Build history of the part. All positions in model axes, mm. A direction names the side the tool comes from. Coordinates: 2 decimals unless noted, no trailing zeros. Write each loop counter-clockwise with the first axis right and the second up, starting at its lowest first coordinate (ties: lowest second). Pieces come first, ordered by that corner, then holes.
```python
from build123d import *

# Parameters (mm, degrees)
BOSS_EXTRUDE1_DEPTH = 5
SKETCH2_W           = 5
SKETCH2_H           = 10
CUT_EXTRUDE1_DEPTH  = 5
SKETCH3_W           = 20
SKETCH3_H           = 20
BOSS_EXTRUDE2_DEPTH = 1
SKETCH5_R           = 5
CUT_EXTRUDE2_DEPTH  = 10
SKETCH6_R           = 5.5
BOSS_EXTRUDE3_DEPTH = 35
SKETCH7_R           = 4
BOSS_EXTRUDE4_DEPTH = 12


# Read off the part's stored shape, not the designer's step: Boss-Extrude1
with BuildPart() as part:
    # Boss-Extrude1 outline → Boss-Extrude1 (new body)
    with BuildSketch(Plane(origin=(0, 0, 0), x_dir=(1, 0, 0), z_dir=(0, 1, 0))):
        with BuildLine():
            ThreePointArc((-68.420925207, 104.11482166), (-83.313400439, 95.590634086), (-89.202352286, 79.47331922))
            Line((-89.202352286, 79.47331922), (-69.202352286, 79.47331922))
            Line((-69.202352286, 79.47331922), (-69.202352286, 31.47331922))
            Line((-69.202352286, 31.47331922), (-89.202352286, 31.47331922))
            Line((-89.202352286, 31.47331922), (-89.202352286, -35))
            Line((-89.202352286, -35), (-74.202352286, -35))
            Line((-74.202352286, -35), (-74.202352286, -85))
            Line((-74.202352286, -85), (-89.202352286, -85))
            ThreePointArc((-89.202352286, -85), (-81.880021816, -102.67766953), (-64.202352286, -110))
            Line((-64.202352286, -110), (65.797647714, -110))
            ThreePointArc((65.797647714, -110), (83.475317244, -102.67766953), (90.797647714, -85))
            Line((90.797647714, -85), (75.797647714, -85))
            Line((75.797647714, -85), (75.797647714, -35))
            Line((75.797647714, -35), (90.797647714, -35))
            Line((90.797647714, -35), (90.797647714, 31.47331922))
            Line((90.797647714, 31.47331922), (70.797647714, 31.47331922))
            Line((70.797647714, 31.47331922), (70.797647714, 79.47331922))
            Line((70.797647714, 79.47331922), (90.797645004, 79.473319219))
            ThreePointArc((90.797645004, 79.473319219), (84.90638671, 95.581731914), (70.020633234, 104.102425978))
            ThreePointArc((70.020633234, 104.102425978), (46.687380596, 107.414128219), (23.202394477, 109.379701262))
            Line((23.202394477, 109.379701262), (23.202394477, 89.994181642))
            Line((23.202394477, 89.994181642), (-24.797605523, 89.994181642))
            Line((-24.797605523, 89.994181642), (-24.797605523, 109.196602404))
            ThreePointArc((-24.797605523, 109.196602404), (-46.677357907, 107.240236017), (-68.420925207, 104.11482166))
        make_face()
    extrude(amount=BOSS_EXTRUDE1_DEPTH)

    # Sketch2 → Cut-Extrude1 (cut)
    with BuildSketch(Plane(origin=(0, 5, 0), x_dir=(1, 0, 0), z_dir=(0, 1, 0))):
        with Locations((3.297647714, -55)):
            Rectangle(SKETCH2_W, SKETCH2_H)
    extrude(amount=-CUT_EXTRUDE1_DEPTH, mode=Mode.SUBTRACT)

    # Sketch3 → Boss-Extrude2 (add)
    with BuildSketch(Plane(origin=(0, 5, 0), x_dir=(1, 0, 0), z_dir=(0, 1, 0))):
        with Locations((45.797647714, 60)):
            Rectangle(SKETCH3_W, SKETCH3_H)
        with Locations((-44.202352286, 60)):
            Rectangle(SKETCH3_W, SKETCH3_H)
    extrude(amount=BOSS_EXTRUDE2_DEPTH)

    # Sketch5 → Cut-Extrude2 (cut)
    with BuildSketch(Plane(origin=(0, 5, 0), x_dir=(1, 0, 0), z_dir=(0, 1, 0))):
        with Locations(Location((-77.202352286, 20, 0), (0, 0, 270))):
            Circle(SKETCH5_R)
        with Locations(Location((-77.202352286, -20, 0), (0, 0, 270))):
            Circle(SKETCH5_R)
        with Locations(Location((-77.202352286, 87.5, 0), (0, 0, 270))):
            Circle(SKETCH5_R)
        with Locations(Location((-77.202352286, -94, 0), (0, 0, 270))):
            Circle(SKETCH5_R)
        with Locations(Location((0, 0, 0), (0, 0, 270))):
            Circle(SKETCH5_R)
        with Locations(Location((77.202352286, -94, 0), (0, 0, 270))):
            Circle(SKETCH5_R)
        with Locations(Location((77.202352286, -20, 0), (0, 0, 270))):
            Circle(SKETCH5_R)
        with Locations(Location((77.202352286, 20, 0), (0, 0, 270))):
            Circle(SKETCH5_R)
        with Locations(Location((77.202352286, 87.5, 0), (0, 0, 270))):
            Circle(SKETCH5_R)
    extrude(amount=-CUT_EXTRUDE2_DEPTH, mode=Mode.SUBTRACT)

    # Sketch6 → Boss-Extrude3 (add)
    with BuildSketch(Plane.XZ):
        with Locations(Location((-77.202352286, 94, 0), (0, 0, 90))):
            Circle(SKETCH6_R)
        with Locations(Location((-77.202352286, 20, 0), (0, 0, 90))):
            Circle(SKETCH6_R)
        with Locations(Location((-77.202352286, -20, 0), (0, 0, 90))):
            Circle(SKETCH6_R)
        with Locations(Location((-77.202352286, -87.5, 0), (0, 0, 90))):
            Circle(SKETCH6_R)
        with Locations(Location((0, 0, 0), (0, 0, 90))):
            Circle(SKETCH6_R)
        with Locations(Location((78.797647714, -87.5, 0), (0, 0, 90))):
            Circle(SKETCH6_R)
        with Locations(Location((78.797647714, -20, 0), (0, 0, 90))):
            Circle(SKETCH6_R)
        with Locations(Location((78.797647714, 20, 0), (0, 0, 90))):
            Circle(SKETCH6_R)
        with Locations(Location((78.797647714, 94, 0), (0, 0, 90))):
            Circle(SKETCH6_R)
    extrude(amount=BOSS_EXTRUDE3_DEPTH)

    # Sketch7 → Boss-Extrude4 (add)
    with BuildSketch(Plane(origin=(0, 5, 0), x_dir=(1, 0, 0), z_dir=(0, 1, 0))):
        with Locations(Location((-50, 0, 0), (0, 0, 270))):
            Circle(SKETCH7_R)
        with Locations(Location((50, 0, 0), (0, 0, 270))):
            Circle(SKETCH7_R)
    extrude(amount=BOSS_EXTRUDE4_DEPTH)


solid = part.part
```
1. Saw through at C-C on y = 11. List the corners of the cut face in (x, z), plus the area to 3 significant figures.
Computed values:
outline: circle Ø8 at (-50, 0); circle Ø8 at (50, 0)
area: 101 mm2
2. Flat gauge pins, fed straight in: pin 1 (1.5 mm diameter, centred on y = 1.5, z = -49.5, fed in from -X); pin 2 (12 mm diameter, centred on y = -9, z = -33, fed in from -X); pin 3 (4 mm diameter, centred on x = -82, y = 1.5, fed in from +Z); pin 4 (1.5 mm diameter, centred on x = 4, y = 1.5, fed in from -Z). Where does each tip first touch, or does it go through?
Computed values:
pin 1: stops at x = -69.2
pin 2: passes through
pin 3: stops at z = 104.38
pin 4: stops at z = -89.99
3. Saw through at A-A on z = 20. List the corners of the cut face in (x, y), plus the area to 3 significant figures.
Computed values:
outline: (-89.2, 0) - (-82.7, 0) - (-82.7, -35) - (-71.7, -35) - (-71.7, 0) - (72.2, 0) - (72.2, 5) - (-72.2, 5) - (-72.2, 0) - (-82.2, 0) - (-82.2, 5) - (-89.2, 5) - close; (73.3, -35) - (84.3, -35) - (84.3, 0) - (90.8, 0) - (90.8, 5) - (82.2, 5) - (82.2, 0) - (73.3, 0) - close
area: 1,570 mm2
4. 3-axis set-ups, long thin cutter, end or side, ignore diameter. For faces 4 (the face through (-52.4, 10.9, -3.2)), 5 (the face through (23.202, 2, -100)), 6 (the face through (74.16, -17.26, 22.96)), 7 (the face through (-82, 2, 85)), 8 (the face through (81, 2, -31.473)): which of +Z, -Z, +X, -X, +Y, -Y reach the whole face in a straight line?
Computed values:
face 4: +Y
face 5: -Z, +Y, -Y
face 6: -Y
face 7: -X, +Y, -Y
face 8: +X, +Y, -Y
5. Mould opens along X. For faces 1 (the face through (70.798, 2, -55)), 2 (the face through (0.798, 3, 55)), 3 (the face through (83, 2, 35)) say: +X half, -X half, draft (parallel to the pull), parting line (faces both ways), or undercut.
Computed values:
face 1: +X half
face 2: undercut
face 3: draft
6. Saw through at D-D on z = 94. List the corners of the cut face in (x, y).
Computed values:
outline: (-87.53, 0) - (-82.7, 0) - (-82.7, -35) - (-71.7, -35) - (-71.7, 0) - (72.2, 0) - (72.2, 5) - (-72.2, 5) - (-72.2, 0) - (-82.2, 0) - (-82.2, 5) - (-87.53, 5) - close; (73.3, -35) - (84.3, -35) - (84.3, 0) - (89.12, 0) - (89.12, 5) - (82.2, 5) - (82.2, 0) - (73.3, 0) - close
7. Saw through at B-B on y = -24. State how many separate pieces and enclosed holes the cut face has, plus the area to 3 significant figures.
Computed values:
separate pieces: 9
enclosed holes: 0
area: 855 mm2
8. Probe line 1 along X through (y, z) = (3, 20); line 2 along X through (y, z) = (3, -87); line 3 along X through (y, z) = (-29, 94). List the from-to ranges inside material, lowest first.
Computed values:
line 1: x = -89.2 to -82.2, -72.2 to 72.2, 82.2 to 90.8
line 2: x = -88.04 to -82.18, -72.23 to 72.23, 82.18 to 89.63
line 3: x = -82.7 to -71.7, 73.3 to 84.3
